The listing builds one solid part. Answer for the finished solid, in the listing's coordinates (mm). Face numbers are marked on the shaded views. A direction names the side the tool comes from. Coordinates: 2 decimals unless noted, no trailing zeros. Order: outer loops, then holes, each group sorted by start corner. A loop starts at its lowest first (then second) coordinate and runs counter-clockwise, first axis right, second up. Notation, with made-up numbers: (67, 34.5) -> (85, 34.5) arc R10 ccw to (85, 45.5) -> close; hole circle Ø7 at (21.25, 87). An arc over 180 degrees is marked (long way). Return JSON: item names as keys, results as strings.
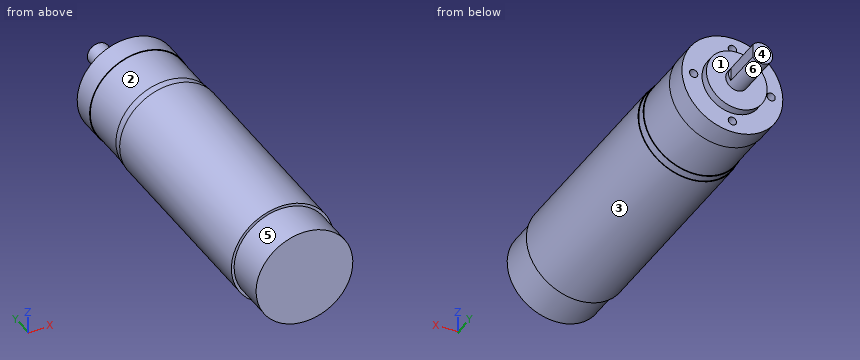
from build123d import *

# Parameters (mm, degrees)
ESQUISSE1_R      = 17.492
EXTRUSION1_DEPTH = 15
ESQUISSE2_R      = 18.491
EXTRUSION2_DEPTH = 76.339
ESQUISSE3_R      = 18.25
EXTRUSION3_DEPTH = 3
ESQUISSE4_R      = 18
EXTRUSION4_DEPTH = 18
ESQUISSE5_R      = 18.241
EXTRUSION5_DEPTH = 8.5
ESQUISSE6_R      = 10.977
EXTRUSION6_DEPTH = 3
ESQUISSE7_R      = 4
EXTRUSION7_DEPTH = 17
ESQUISSE8_W      = 2.691612919
ESQUISSE8_H      = 12.532822653
EXTRUSION8_DEPTH = 15
ESQUISSE9_R      = 1.5
EXTRUSION9_DEPTH = 7


with BuildPart() as part:
    # Esquisse1 → Extrusion1 (new body)
    with BuildSketch(Plane(origin=(0, 0, 0), x_dir=(1, 0, 0), z_dir=(0, 1, 0))):
        with Locations(Location((0, 0, 0), (0, 0, 270))):
            Circle(ESQUISSE1_R)
    extrude(amount=EXTRUSION1_DEPTH)

    # Esquisse2 → Extrusion2 (add)
    with BuildSketch(Plane(origin=(0, 15, 0), x_dir=(1, 0, 0), z_dir=(0, 1, 0))):
        with Locations(Location((0, 0, 0), (0, 0, 270))):
            Circle(ESQUISSE2_R)
    extrude(amount=EXTRUSION2_DEPTH)

    # Esquisse3 → Extrusion3 (add)
    with BuildSketch(Plane(origin=(0, 91.339, 0), x_dir=(1, 0, 0), z_dir=(0, 1, 0))):
        with Locations(Location((0, 0, 0), (0, 0, 270))):
            Circle(ESQUISSE3_R)
    extrude(amount=EXTRUSION3_DEPTH)

    # Esquisse4 → Extrusion4 (add)
    with BuildSketch(Plane(origin=(0, 94.339, 0), x_dir=(1, 0, 0), z_dir=(0, 1, 0))):
        with Locations(Location((0, 0, 0), (0, 0, 270))):
            Circle(ESQUISSE4_R)
    extrude(amount=EXTRUSION4_DEPTH)

    # Esquisse5 → Extrusion5 (add)
    with BuildSketch(Plane(origin=(0, 112.339, 0), x_dir=(1, 0, 0), z_dir=(0, 1, 0))):
        with Locations(Location((0, 0, 0), (0, 0, 270))):
            Circle(ESQUISSE5_R)
    extrude(amount=EXTRUSION5_DEPTH)

    # Esquisse6 → Extrusion6 (add)
    with BuildSketch(Plane(origin=(0, 120.839, 0), x_dir=(1, 0, 0), z_dir=(0, 1, 0))):
        with Locations(Location((0, 0, 0), (0, 0, 270))):
            Circle(ESQUISSE6_R)
    extrude(amount=EXTRUSION6_DEPTH)

    # Esquisse7 → Extrusion7 (add)
    with BuildSketch(Plane(origin=(0, 123.839, 0), x_dir=(-1, 0, 0), z_dir=(0, 1, 0))):
        with Locations(Location((0, 0, 0), (0, 0, 90))):
            Circle(ESQUISSE7_R)
    extrude(amount=EXTRUSION7_DEPTH)

    # Esquisse8 → Extrusion8 (cut)
    with BuildSketch(Plane(origin=(0, 140.839, 0), x_dir=(1, 0, 0), z_dir=(0, 1, 0))):
        with Locations((4.55780646, -1.030383071)):
            Rectangle(ESQUISSE8_W, ESQUISSE8_H)
    extrude(amount=-EXTRUSION8_DEPTH, mode=Mode.SUBTRACT)

    # Esquisse9 → Extrusion9 (cut)
    with BuildSketch(Plane(origin=(0, 120.839, 0), x_dir=(1, 0, 0), z_dir=(0, 1, 0))):
        with Locations(Location((0, 14, 0), (0, 0, 270))):
            Circle(ESQUISSE9_R)
        with Locations(Location((14.001, 0.001, 0), (0, 0, 270))):
            Circle(ESQUISSE9_R)
        with Locations(Location((0.002, -14, 0), (0, 0, 270))):
            Circle(ESQUISSE9_R)
        with Locations(Location((-13.999, -0.001, 0), (0, 0, 270))):
            Circle(ESQUISSE9_R)
    extrude(amount=-EXTRUSION9_DEPTH, mode=Mode.SUBTRACT)


solid = part.part
1. The part is cut by section D-D on y = 36. Give the vertices of the cut face in (x, z), and give its area (3 significant figures).
Answer block:
{"outline": "circle Ø36.98 at (0, 0)", "area": "1,070 mm2"}
2. Each of these flat-tipped pins is pushed along its axis until it touches: pin 1 Ø8 at (x, z) = (4.5, -8) entering from +Y; pin 2 Ø1 at (x, y) = (-6, 50.5) entering from +Z; pin 3 Ø4 at (x, z) = (-4.5, 13.5) entering from +Y. Where does it stop, or does it pass through?
Answer block:
{"pin 1": "stops at y = 123.84", "pin 2": "stops at z = 17.65", "pin 3": "stops at y = 120.84"}
3. For the marked faces 4, 5 and 6, determine the directions among +Z, -Z, +X, -X, +Y, -Y from which every point of the face is accessible in a straight line to the end or side of a thin tool.
Answer block:
{"face 4": "+Z, -Z, +X, -X, +Y", "face 5": "-Y", "face 6": "+Y"}
4. Consider line 1 (Y direction, x = -9, z = 16); line 2 (Y direction, x = 9, z = 7); line 3 (X direction, y = 117, z = 14). Determine where each line is inside the solid, lowest interval first. Write a range as from..to.
Answer block:
{"line 1": "y = 15..91.34", "line 2": "y = 0..120.84", "line 3": "x = -11.69..-1.5, 1.5..11.69"}
5. The part is cut by section C-C on x = 6. Give the vertices of the cut face in (y, z).
Answer block:
{"outline": "(0, -16.43) -> (15, -16.43) -> (15, -17.49) -> (91.34, -17.49) -> (91.34, -17.24) -> (94.34, -17.24) -> (94.34, -16.97) -> (112.34, -16.97) -> (112.34, -17.23) -> (120.84, -17.23) -> (120.84, -9.19) -> (123.84, -9.19) -> (123.84, 9.19) -> (120.84, 9.19) -> (120.84, 17.23) -> (112.34, 17.23) -> (112.34, 16.97) -> (94.34, 16.97) -> (94.34, 17.24) -> (91.34, 17.24) -> (91.34, 17.49) -> (15, 17.49) -> (15, 16.43) -> (0, 16.43) -> close"}
6. The part is cut by section B-B on z = -14. Give the vertices of the cut face in (x, y), and give its area (3 significant figures).
Answer block:
{"outline": "(-12.08, 15) -> (-10.49, 15) -> (-10.49, 0) -> (10.49, 0) -> (10.49, 15) -> (12.08, 15) -> (12.08, 91.34) -> (11.71, 91.34) -> (11.71, 94.34) -> (11.31, 94.34) -> (11.31, 112.34) -> (11.69, 112.34) -> (11.69, 120.84) -> (1.5, 120.84) -> (1.5, 113.84) -> (-1.5, 113.84) -> (-1.5, 120.84) -> (-11.69, 120.84) -> (-11.69, 112.34) -> (-11.31, 112.34) -> (-11.31, 94.34) -> (-11.71, 94.34) -> (-11.71, 91.34) -> (-12.08, 91.34) -> close", "area": "2,810 mm2"}
7. The part is cut by section A-A on y = 96. Give the vertices of the cut face in (x, z).
Answer block:
{"outline": "circle Ø36 at (0, 0)"}
8. Determine the mould class of the marked faces 1, 2 and 3 for opening direction Y: pulls with the +Y half, pulls with the -Y half, needs draft (parallel to the pull), parting line crosses it, or undercut.
Answer block:
{"face 1": "pulls with the +Y half", "face 2": "undercut", "face 3": "needs draft"}
